Geometry check sheet. Reference: the model listing, model coordinates, mm. A direction names the side the tool comes from. Round coordinates to 2 decimals unless told otherwise and drop trailing zeros. Order: outer loops, then holes, each group sorted by start corner. A loop starts at its lowest first (then second) coordinate and runs counter-clockwise, first axis right, second up. Notation, with made-up numbers: (-14.5, 1) -> (10.5, 1) arc R13 cw to (10.5, 8) -> close; hole circle Ø11 at (50.25, 68). An arc over 180 degrees is marked (long way). Use a Markdown table: item, result. Add a question column.
Item 1: Sectioned sample at D-D, the plane z = -34. Record the cut outline in (x, y), and give its area (3 significant figures).
Item 2: Sectioned sample at A-A, the plane z = -27.5. Record the cut outline in (x, y), and give its area (3 significant figures).
Item 3: Set-up check for faces 4 (the cylindrical face through (-64.456, -1.479, -25.794)), 5 (the flat face through (-39.016, 1, -26)): record each of +Z, -Z, +X, -X, +Y, -Y from which the full face is reachable in a straight line by a thin tool's end or side.
Item 4: Mould release check, pull along Z, two halves, no side actions. Record for faces 1 (the cylindrical face through (-90.16, 1.01, -2.74)), 2 (the flat face through (-64.3, -3, -27.8)), 3 (the flat face through (-62, 0, -26)): pulls with the +Z half, pulls with the -Z half, needs draft (parallel to the pull), parting line crosses it, or undercut.
Item 5: Sectioned sample at B-B, the plane x = -73. Record the cut outline in (y, z), and give its area (3 significant figures).
Item 6: Sectioned sample at C-C, the plane y = -2.4. Record the cut outline in (x, z), and give its area (3 significant figures).
Item 7: Material ranges on probe 1 along Y at (x, z) = (-44, -44); probe 2 along Z at (x, y) = (-61.5, -2.8); probe 3 along Z at (x, y) = (-64, -1.85), recorded low to high. Write a range as [from, to].
Item 8: Gauge pin test, flat ends, axial feed: pin 1 Ø2.5 at (x, z) = (-63, -26.5) entering from -Y; pin 2 Ø14.5 at (x, z) = (-54.5, -25.5) entering from -Y. Record the tip position at first contact, or that the pin passes through.
from build123d import *

# Parameters (mm, degrees)
SKETCH3_W           = 52
SKETCH3_H           = 49
BOSS_EXTRUDE3_DEPTH = 2
SKETCH5_R           = 3.5
SKETCH5_R_2         = 2.5
BOSS_EXTRUDE5_DEPTH = 3
FILLET1_R           = 3


with BuildPart() as part:
    # Sketch3 → Boss-Extrude3 (new body)
    with BuildSketch(Plane(origin=(0, 0, 0), x_dir=(1, 0, 0), z_dir=(0, 1, 0))):
        with Locations((-65.015948434, 26.335900173)):
            Rectangle(SKETCH3_W, SKETCH3_H)
    extrude(amount=BOSS_EXTRUDE3_DEPTH)

    # Sketch5 → Boss-Extrude5 (add)
    with BuildSketch(Plane.XZ):
        with Locations(Location((-62.015948434, -26.335900173, 0), (0, 0, 270))):
            Circle(SKETCH5_R)
        with Locations(Location((-62.015948434, -26.335900173, 0), (0, 0, 270))):
            Circle(SKETCH5_R_2, mode=Mode.SUBTRACT)
    extrude(amount=BOSS_EXTRUDE5_DEPTH)

    # Fillet1
    fillet1_edges = [part.edges().sort_by_distance(p)[0] for p in [
        (-39.015948434, 1, -50.835900173),
        (-39.015948434, 1, -1.835900173),
        (-91.015948434, 1, -1.835900173),
        (-91.015948434, 1, -50.835900173),
    ]]
    fillet(fillet1_edges, radius=FILLET1_R)


solid = part.part
Found:
| question | item | result |
|---|---|---|
| 1 | outline | (-91.02, 0) -> (-39.02, 0) -> (-39.02, 2) -> (-91.02, 2) -> close |
| 1 | area | 104 mm2 |
| 2 | outline | (-91.02, 0) -> (-65.32, 0) -> (-65.32, -3) -> (-64.23, -3) -> (-64.23, 0) -> (-59.8, 0) -> (-59.8, -3) -> (-58.72, -3) -> (-58.72, 0) -> (-39.02, 0) -> (-39.02, 2) -> (-91.02, 2) -> close |
| 2 | area | 111 mm2 |
| 3 | face 4 | -Y |
| 3 | face 5 | +Z, -Z, +X, +Y, -Y |
| 4 | face 1 | pulls with the +Z half |
| 4 | face 2 | needs draft |
| 4 | face 3 | undercut |
| 5 | outline | (0, -50.84) -> (2, -50.84) -> (2, -1.84) -> (0, -1.84) -> close |
| 5 | area | 98.0 mm2 |
| 6 | outline | circle Ø7 at (-62.02, -26.34); hole circle Ø5 at (-62.02, -26.34) |
| 6 | area | 18.8 mm2 |
| 7 | probe 1 | y = [0, 2] |
| 7 | probe 2 | z = [-29.8, -28.78], [-23.89, -22.87] |
| 7 | probe 3 | z = [-29.22, -27.86], [-24.81, -23.45] |
| 8 | pin 1 | stops at y = 0 |
| 8 | pin 2 | stops at y = -3 |
